```python
from build123d import *

# Parameters (mm, degrees)
SKETCH1_R           = 7.5
BOSS_EXTRUDE1_DEPTH = 250
SKETCH2_R           = 5
CUT_EXTRUDE1_DEPTH  = 10
SKETCH3_R           = 9.435011435
SKETCH3_R_2         = 5
CUT_EXTRUDE2_DEPTH  = 19
SKETCH5_R           = 25.765699078
CUT_EXTRUDE3_DEPTH  = 221
SKETCH6_R           = 5.5
BOSS_EXTRUDE2_DEPTH = 10


with BuildPart() as part:
    # Sketch1 → Boss-Extrude1 (new body)
    with BuildSketch(Plane.XY):
        Circle(SKETCH1_R)
    extrude(amount=BOSS_EXTRUDE1_DEPTH)

    # Sketch2 → Cut-Extrude1 (cut)
    with BuildSketch(Plane.XY):
        Circle(SKETCH2_R)
    extrude(amount=CUT_EXTRUDE1_DEPTH, mode=Mode.SUBTRACT)

    # Sketch3 → Cut-Extrude2 (cut)
    with BuildSketch(Plane(origin=(0, 0, 10), x_dir=(-1, 0, 0), z_dir=(0, 0, -1))):
        Circle(SKETCH3_R)
        Circle(SKETCH3_R_2, mode=Mode.SUBTRACT)
    extrude(amount=-CUT_EXTRUDE2_DEPTH, mode=Mode.SUBTRACT)


with BuildPart() as cut_extrude2_piece_1:
    # of the separate pieces the step leaves, piece 1, a body of its own (cut_extrude2_pieces)
    add(part.part.solids().sort_by_distance((7.5, 0, 29))[0])

    # Sketch5 → Cut-Extrude3 (cut)
    with BuildSketch(Plane(origin=(0, 0, 29), x_dir=(-1, 0, 0), z_dir=(0, 0, -1))):
        Circle(SKETCH5_R)
    extrude(amount=-CUT_EXTRUDE3_DEPTH, mode=Mode.SUBTRACT)



with BuildPart() as cut_extrude2_piece_2:
    # of the separate pieces the step leaves, piece 2, a body of its own (cut_extrude2_pieces)
    add(part.part.solids().sort_by_distance((7.5, 0, 0))[0])


with BuildPart() as cut_extrude2_piece_1_1:
    add(cut_extrude2_piece_1.part)

    add(cut_extrude2_piece_2.part)  # Boss-Extrude2 merges Cut-Extrude2 piece 2
    # Sketch6 → Boss-Extrude2 (add)
    with BuildSketch(Plane(origin=(0, 0, 10), x_dir=(-1, 0, 0), z_dir=(0, 0, -1))):
        Circle(SKETCH6_R)
    extrude(amount=BOSS_EXTRUDE2_DEPTH)


solid = cut_extrude2_piece_1_1.part
```
Part model, mm, in its own coordinate system. A direction names the side the tool comes from. Give positions to 0.01 mm unless a question says otherwise; leave off trailing zeros. Order: outer loops, then holes, each group sorted by start corner. A loop starts at its lowest first (then second) coordinate and runs counter-clockwise, first axis right, second up. Notation, with made-up numbers: (55.5, 2.25) - (77.5, 2.25) arc R13 cw to (77.5, 14.25) - close; hole circle Ø11 at (24.25, 53.25). An arc over 180 degrees is marked (long way). Use one line per item in the form item = value.
Item 1: Slice it at D-D on y = 6. Give the cut face in (x, z), and give its area (3 significant figures).
Solution:
outline = (-4.5, 0) - (4.5, 0) - (4.5, 10) - (-4.5, 10) - close
area = 90.0 mm2
Item 2: Slice it at C-C on z = 27. Give the cut face in (x, y).
Solution:
outline = circle Ø10 at (0, 0)
Item 3: Slice it at A-A on y = 0. Give the cut face in (x, z), and give its area (3 significant figures).
Solution:
outline = (-7.5, 0) - (7.5, 0) - (7.5, 10) - (5, 10) - (5, 29) - (-5, 29) - (-5, 10) - (-7.5, 10) - close
area = 340 mm2
Item 4: Which spindle directions (+Z, -Z, +X, -X, +Y, -Y) get a long thin tool onto all of the face, cutting with end or side? Do faces 1 (the face through (-2, -5, 10)), 2 (the face through (0, 0, 29)). Say none if no direction does.
Solution:
face_1 = +Z
face_2 = +Z, +X, -X, +Y, -Y
Item 5: Pin check, flat tips, straight feed: pin 1 Ø5 at (x, z) = (1, 13.5) entering from +Y; pin 2 Ø1.5 at (x, z) = (-3, 8) entering from +Y; pin 3 Ø6 at (y, z) = (4.5, 7) entering from +X. Stop position of each tip, or through.
Solution:
pin_1 = 5
pin_2 = 7.15
pin_3 = 7.35
Item 6: Probe probe 1 along Z at (x, y) = (-6.25, -1.25); probe 2 along Y at (x, z) = (-2.25, 8.75); probe 3 along Y at (x, z) = (-3.25, 6). List the from-to ranges inside material, lowest first. Write a range as from..to.
Solution:
probe_1 = 0..10
probe_2 = -7.15..7.15
probe_3 = -6.76..6.76
